For this review, take the finished solid that the model builds, in its own axes (mm). A direction names the side the tool comes from. Coordinates: 2 decimals unless noted, no trailing zeros. Order: outer loops, then holes, each group sorted by start corner. A loop starts at its lowest first (then second) coordinate and runs counter-clockwise, first axis right, second up. Notation, with made-up numbers: (0, 75) -> (27, 75) arc R35 ccw to (27, 108) -> close; hole circle Ø7 at (34, -9). An arc over 180 degrees is marked (long way). Write item = value, one per line. Start each with the question number.
1) Insertion check: pin 1 Ø1.5 at (x, y) = (2, -3) entering from +Z; pin 2 Ø1 at (x, y) = (-2, -3) entering from +Z. Each pin has a flat end and moves straight along its axis. Give the tip position at first contact, or say it passes through.
2) Wall thickness on probe 1 along X at (y, z) = (0, -25.3); probe 2 along X at (y, z) = (0, -5.25): over which ranges is each line inside the solid? List them lowest first. Write a range as [from, to].
3) Machinability: for faces 4 (the face through (-1, -3, -21)), 5 (the face through (0.867, -3.905, -16.07)), 6 (the face through (0.748, 0.976, -3.955)), which of the approach directions +Z, -Z, +X, -X, +Y, -Y give a long, thin tool a straight path to every point of the face, cutting with its end or side? Answer none if there is none.
4) Consider section A-A on z = -5.25. Give the boundary of the cut face in (x, y).
5) Consider section D-D on z = -10.5. Give the boundary of the cut face in (x, y).
6) Consider section B-B on x = 1.75. Give the boundary of the cut face in (y, z), and give its area (3 significant figures).
7) Draft analysis for pull direction X (two halves, no side actions). For faces 1 (the face through (-1, -1, 0)), 2 (the face through (3, 0, -8)), 3 (the face through (-0.07, -1.5, -24.63)), state which applies: +X half, -X half, draft (parallel to the pull), parting line (faces both ways), or undercut.
Autodesk Inventor part; units mm, degrees
ref_plane "YZ Plane" through (0, 0, 0) normal (1, 0, 0) x (0, 1, 0)
ref_plane "XZ Plane" through (0, 0, 0) normal (0, 1, 0) x (-1, 0, 0)
ref_plane "XY Plane" through (0, 0, 0) normal (0, 0, 1) x (1, 0, 0)
sketch "Sketch1" plane through (0, 0, 0) normal (0, 1, 0) x (-1, 0, 0)
  line L0 (0, 0) -> (2.5, 0)
  line L1 (2.5, 0) -> (2.5, -26.2)
  line L2 (2.5, -26.2) -> (0, -26.2)
  line L3 (0, -26.2) -> (0, 0)
  line L4 (2.5, -5.8) -> (3, -5.8)
  line L5 (3, -5.8) -> (3, -11)
  line L6 (3, -11) -> (4, -11)
  line L7 (4, -11) -> (4, -21)
  line L8 (4, -21) -> (3, -21)
  line L9 (3, -21) -> (3, -26.2)
  line L10 (3, -26.2) -> (2.5, -26.2)
  dimension "d0" = 5
  dimension "d10" = 6
  dimension "d11" = 5.8
  dimension "d12" = 8
  dimension "d13" = 5.2
  dimension "d14" = 5.2
  dimension "d15" = 10
revolve "Revolution1" add sketch "Sketch1" angle 360 about axis through (0, 0, -26.2) along (0, 0, 1)
sketch "Sketch2" plane through (0, 0, 0) normal (0, 0, 1) x (1, 0, 0)
  point P0 (0, 0)
  point P1 (0, 0)
hole "Hole1" at (0, 0, 0) direction (0, 0, -1) diameter 2.459 depth 7.8 tip angle 118
sketch "Sketch3" plane through (0, 0, -26.2) normal (0, 0, -1) x (-1, 0, 0)
  circle A0 centre (0, 0) radius 1.2295
  point P0 (0, 0)
hole "Hole2" at (0, 0, -26.2) direction (0, 0, 1) diameter 3 depth 3.1 tip angle 118
equation "\"d14\" = d13"
properties part number "TorquimeterShaft" material "Stainless Steel, Austenitic"
Answer sheet:
q1.pin_1 = -5.8
q1.pin_2 = -11
q2.probe_1 = [-3, -1.5], [1.5, 3]
q2.probe_2 = [-2.5, -1.23], [1.23, 2.5]
q3.face_4 = -Z
q3.face_5 = +Z, -Z
q3.face_6 = +Z
q4.outline = circle Ø5 at (0, 0); hole circle Ø2.46 at (0, 0)
q5.outline = circle Ø6 at (0, 0)
q6.outline = (-3.6, -21) -> (-2.44, -21) -> (-2.44, -26.2) -> (2.44, -26.2) -> (2.44, -21) -> (3.6, -21) -> (3.6, -11) -> (2.44, -11) -> (2.44, -5.8) -> (1.79, -5.8) -> (1.79, 0) -> (-1.79, 0) -> (-1.79, -5.8) -> (-2.44, -5.8) -> (-2.44, -11) -> (-3.6, -11) -> close
q6.area = 143 mm2
q7.face_1 = draft
q7.face_2 = parting line
q7.face_3 = undercut
